Autodesk Inventor part; units mm, degrees
ref_plane "YZ Plane" through (0, 0, 0) normal (1, 0, 0) x (0, 1, 0)
ref_plane "XZ Plane" through (0, 0, 0) normal (0, 1, 0) x (-1, 0, 0)
ref_plane "XY Plane" through (0, 0, 0) normal (0, 0, 1) x (1, 0, 0)
sketch "Sketch1" plane through (0, 0, 0) normal (1, 0, 0) x (0, 1, 0)
  line L0 (0, 0) -> (-3.175, 0)
  line L1 (-3.175, 0) -> (-3.175, -50.8)
  line L2 (-3.175, -50.8) -> (0, -50.8)
  line L3 (0, -50.8) -> (0, 0)
  line L4 (-3.175, -50.8) -> (98.425, -50.8)
  line L5 (98.425, -50.8) -> (98.425, -53.975)
  line L6 (98.425, -53.975) -> (-3.175, -53.975)
  line L7 (-3.175, -53.975) -> (-3.175, -50.8)
  dimension "d0" = 3.175
  dimension "d1" = 50.8
  dimension "d2" = 101.6
  dimension "d3" = 3.175
extrude "Extrusion1" add sketch "Sketch1" along normal blind 50.8
sketch "Sketch2" plane through (0, 0, -50.8) normal (0, 0, 1) x (1, 0, 0)
  circle A0 centre (25.4, 76.2) radius 8.509
  line L0 (0, 98.425) -> (0, 0)
  line L1 (0, 0) -> (50.8, 0)
  dimension "d6" = 17.018
  dimension "d7" = 25.4
  dimension "d8" = 76.2
extrude "Extrusion2" cut sketch "Sketch2" against normal through all
fillet "Fillet1" radius 25.4 2 edges at (50.8, 98.425, -52.3875) (0, 98.425, -52.3875)
properties part number "L Connector Ramp" material "Aluminum 6061"
Design review of the part built by this model. Coordinates are the model's own, in mm. A direction names the side the tool comes from. Coordinates: 2 decimals unless noted, no trailing zeros. Order: outer loops, then holes, each group sorted by start corner. A loop starts at its lowest first (then second) coordinate and runs counter-clockwise, first axis right, second up.
1) Take a section at D-D, the plane z = -22.5. Give the boundary of the cut face in (x, y) (3 decimals).
2) Mouldability with a two-part tool opening along X and no side actions: class faces 3 (the cylindrical face through (23.555, 67.893, -52.365)), 4 (the cylindrical face through (7.243, 90.787, -52.41)), 5 (the flat face through (25, -2, 0)) as +X half, -X half, draft (parallel to the pull), parting line (faces both ways), or undercut.
3) Wall thickness on line 1 along Y through (x, z) = (25, -52) (3 decimals); line 2 along Z through (x, y) = (14, 63) (3 decimals); line 3 along Y through (x, z) = (35.5, -16.5) (3 decimals): over which ranges is each line inside the solid? List them lowest first.
4) For faces 1 (the flat face through (25, 0, -26)), 2 (the flat face through (25, -3.175, -27)), list the 3-axis set-ups (+Z, -Z, +X, -X, +Y, -Y) from which the entire face can be reached by the end or side of a thin tool; tool diameter is ignored.
5) Take a section at A-A, the plane x = 22.5. Give the boundary of the cut face in (y, z) (3 decimals), and give its area (3 significant figures).
6) Take a section at B-B, the plane y = 76.2. Give the boundary of the cut face in (x, z) (3 decimals).
7) Clearance check with flat-ended pins moving along their axes: pin 1 (8 mm diameter, centred on y = 35.5, z = -43.5, fed in from -X); pin 2 (15 mm diameter, centred on x = 22.5, z = -22.5, fed in from +Y); pin 3 (3 mm diameter, centred on x = 26.5, y = 26.5, fed in from +Z). State where each tip first meets the part, or that it passes through.
8) Take a section at C-C, the plane y = 15.5. Give the boundary of the cut face in (x, z) (3 decimals).
Returned:
1. outline: (0, -3.175) - (50.8, -3.175) - (50.8, 0) - (0, 0) - close
2. face 3: undercut
2. face 4: -X half
2. face 5: draft
3. line 1: y = -3.175 to 67.7, 84.7 to 98.422
3. line 2: z = -53.975 to -50.8
3. line 3: y = -3.175 to 0
4. face 1: +Z, +X, -X, +Y
4. face 2: +Z, -Z, +X, -X, -Y
5. outline: (-3.175, -53.975) - (68.2, -53.975) - (68.2, -50.8) - (0, -50.8) - (0, 0) - (-3.175, 0) - close; (84.2, -53.975) - (98.259, -53.975) - (98.259, -50.8) - (84.2, -50.8) - close
5. area: 433 mm2
6. outline: (0.199, -53.975) - (16.891, -53.975) - (16.891, -50.8) - (0.199, -50.8) - close; (33.909, -53.975) - (50.601, -53.975) - (50.601, -50.8) - (33.909, -50.8) - close
7. pin 1: passes through
7. pin 2: stops at y = 0
7. pin 3: stops at z = -50.8
8. outline: (0, -53.975) - (50.8, -53.975) - (50.8, -50.8) - (0, -50.8) - close
